```python
from build123d import *

# Parameters (mm, degrees)
F0_W     = 80
F0_H     = 80
F1_DEPTH = 10
F2_R     = 5
F3_W     = 29.726662
F3_H     = 8.11574
F4_DEPTH = 5


with BuildPart() as f1:
    # F0 (on Top) → F1 (new body)
    with BuildSketch(Plane.XY):
        with Locations((-29.271951, -16.949144)):
            Rectangle(F0_W, F0_H)
    extrude(amount=F1_DEPTH)

    # F2
    f2_edges = [f1.edges().sort_by_distance(p)[0] for p in [
        (-69.271951, 23.050856, 5),
        (-69.271951, -56.949144, 5),
        (10.728049, -56.949144, 5),
        (10.728049, 23.050856, 5),
    ]]
    fillet(f2_edges, radius=F2_R)

    # F3 (on face) → F4 (cut)
    with BuildSketch(Plane.XY.offset(10)):
        with Locations((-30.946564, 4.05787)):
            Rectangle(F3_W, F3_H)
    extrude(amount=-F4_DEPTH, mode=Mode.SUBTRACT)


solid = f1.part
```
For this review, take the finished solid that the model builds, in its own axes (mm). A direction names the side the tool comes from. Round coordinates to 2 decimals unless told otherwise and drop trailing zeros. Write each loop counter-clockwise with the first axis right and the second up, starting at its lowest first coordinate (ties: lowest second). Pieces come first, ordered by that corner, then holes. Notation, with made-up numbers: (48.5, 18.5) - (79.5, 18.5) arc R22 ccw to (79.5, 32.5) - close; hole circle Ø9 at (3.5, 82). An arc over 180 degrees is marked (long way). Answer as a JSON object with one key per item and string values.
1. We need section B-B on x = -22.5. Give the boundary of the cut face in (y, z).
Response values:
{"outline": "(-56.95, 0) - (23.05, 0) - (23.05, 10) - (8.12, 10) - (8.12, 5) - (0, 5) - (0, 10) - (-56.95, 10) - close"}
2. We need section A-A on z = 7.25. Give the boundary of the cut face in (x, y).
Response values:
{"outline": "(-69.27, -51.95) arc R5 ccw to (-64.27, -56.95) - (5.73, -56.95) arc R5 ccw to (10.73, -51.95) - (10.73, 18.05) arc R5 ccw to (5.73, 23.05) - (-64.27, 23.05) arc R5 ccw to (-69.27, 18.05) - close; hole (-45.81, 0) - (-16.08, 0) - (-16.08, 8.12) - (-45.81, 8.12) - close"}
3. To check wall thickness, follow line 1 along X through (y, z) = (2, 7); line 2 along Y through (x, z) = (-41.5, 9.75); line 3 along Y through (x, z) = (-65.5, 4.5). State the ranges of each line that lie inside material, in increasing order.
Response values:
{"line 1": "x = -69.27 to -45.81, -16.08 to 10.73", "line 2": "y = -56.95 to 0, 8.12 to 23.05", "line 3": "y = -56.8 to 22.9"}
4. For pin 1 Ø2.5 at (x, y) = (-35, 6) entering from +Z; pin 2 Ø1.5 at (x, y) = (-57, 6) entering from -Z, all flat-tipped, find the tip position at first contact; note any pin that passes through.
Response values:
{"pin 1": "stops at z = 5", "pin 2": "stops at z = 0"}
5. Tool access review of faces 5 (the face through (-45.81, 4, 8)), 6 (the face through (10.728, -17, 5)): name each direction out of +Z, -Z, +X, -X, +Y, -Y from which nothing blocks a thin tool from reaching the whole face with its end or side.
Response values:
{"face 5": "+Z", "face 6": "+Z, -Z, +X, +Y, -Y"}
6. Draft analysis for pull direction Y (two halves, no side actions). For faces 1 (the face through (-31, 8.116, 8)), 2 (the face through (9.224, -55.523, 5.07)), 3 (the face through (-16.083, 4, 8)), 4 (the face through (-30, 23.051, 5)), state which applies: +Y half, -Y half, draft (parallel to the pull), parting line (faces both ways), or undercut.
Response values:
{"face 1": "undercut", "face 2": "-Y half", "face 3": "undercut", "face 4": "+Y half"}
